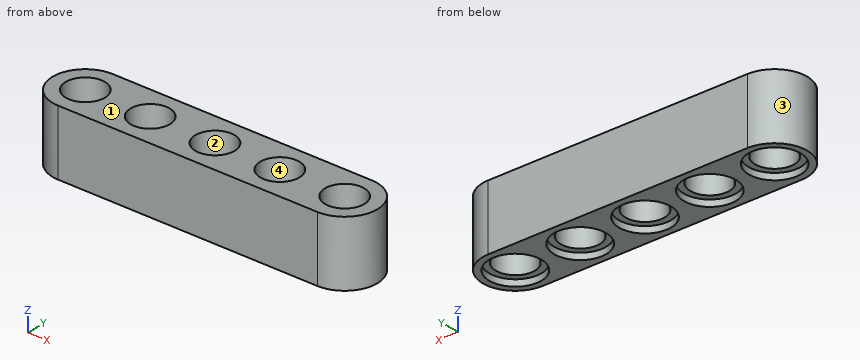
from build123d import *

# Parameters (mm, degrees)
SKETCH_R     = 2.4
PAD_DEPTH    = 8
SKETCH001_R  = 3.2
POCKET_DEPTH = 0.8


with BuildPart() as part:
    # Sketch → Pad (new body)
    with BuildSketch(Plane.XY):
        with BuildLine():
            ThreePointArc((-16, 4), (-20, 0), (-16, -4))
            Line((-16, -4), (16, -4))
            ThreePointArc((16, -4), (20, 0), (16, 4))
            Line((16, 4), (-16, 4))
        make_face()
        with Locations((-16, 0)):
            Circle(SKETCH_R, mode=Mode.SUBTRACT)
        with Locations((16, 0)):
            Circle(SKETCH_R, mode=Mode.SUBTRACT)
        with Locations((8, 0)):
            Circle(SKETCH_R, mode=Mode.SUBTRACT)
        with Locations((-8, 0)):
            Circle(SKETCH_R, mode=Mode.SUBTRACT)
        Circle(SKETCH_R, mode=Mode.SUBTRACT)
    extrude(amount=PAD_DEPTH)

    # Sketch001 → Pocket (cut)
    with BuildSketch(Plane.XY):
        Circle(SKETCH001_R)
        with Locations((-16, 0)):
            Circle(SKETCH001_R)
        with Locations((-8, 0)):
            Circle(SKETCH001_R)
        with Locations((8, 0)):
            Circle(SKETCH001_R)
        with Locations((16, 0)):
            Circle(SKETCH001_R)
    extrude(amount=POCKET_DEPTH, mode=Mode.SUBTRACT)


solid = part.part
Design review of the part built by this model. Coordinates are the model's own, in mm. Face numbers are marked on the shaded views. Round coordinates to 2 decimals unless told otherwise and drop trailing zeros. Write each loop counter-clockwise with the first axis right and the second up, starting at its lowest first coordinate (ties: lowest second). Pieces come first, ordered by that corner, then holes.
Item 1: For pin 1 Ø1.9 at (x, y) = (16, 1.5) entering from -Z; pin 2 Ø3 at (x, y) = (9.5, 1.5) entering from -Z, all flat-tipped, find the tip position at first contact; note any pin that passes through.
Item 2: Wall thickness on L1, parallel to X at y = 0, z = 3.25; L2, parallel to Y at x = 16, z = 4.5; L3, parallel to X at y = 0.5, z = 6.75: over which ranges is each line inside the solid? List them lowest first.
Item 3: Consider section B-B on z = 3.25. Give the boundary of the cut face in (x, y).
Item 4: Consider section A-A on x = 0. Give the boundary of the cut face in (y, z), and give its area (3 significant figures).
Item 5: Consider section D-D on x = 17.5. Give the boundary of the cut face in (y, z).
Item 6: Consider section C-C on y = 0. Count the separate pieces of the cut face and the enclosed holes in it, and give its area (3 significant figures).
Item 7: Draft analysis for pull direction Y (two halves, no side actions). For the marked faces 1, 2, 3 and 4, state which applies: released by +Y, released by -Y, zero draft, split by the parting line, or undercut.
Check values:
1. pin 1: stops at z = 0.8
1. pin 2: stops at z = 0
2. L1: x = -20 to -18.4, -13.6 to -10.4, -5.6 to -2.4, 2.4 to 5.6, 10.4 to 13.6, 18.4 to 20
2. L2: y = -4 to -2.4, 2.4 to 4
2. L3: x = -19.97 to -18.35, -13.65 to -10.35, -5.65 to -2.35, 2.35 to 5.65, 10.35 to 13.65, 18.35 to 19.97
3. outline: (-16, -4) - (16, -4) arc R4 ccw to (16, 4) - (-16, 4) arc R4 ccw to start; hole circle Ø4.8 at (-16, 0); hole circle Ø4.8 at (-8, 0); hole circle Ø4.8 at (0, 0); hole circle Ø4.8 at (8, 0); hole circle Ø4.8 at (16, 0)
4. outline: (-4, 0) - (-3.2, 0) - (-3.2, 0.8) - (-2.4, 0.8) - (-2.4, 8) - (-4, 8) - close; (2.4, 0.8) - (3.2, 0.8) - (3.2, 0) - (4, 0) - (4, 8) - (2.4, 8) - close
4. area: 24.3 mm2
5. outline: (-3.71, 0) - (-2.83, 0) - (-2.83, 0.8) - (-1.87, 0.8) - (-1.87, 8) - (-3.71, 8) - close; (1.87, 0.8) - (2.83, 0.8) - (2.83, 0) - (3.71, 0) - (3.71, 8) - (1.87, 8) - close
6. separate pieces: 6
6. enclosed holes: 0
6. area: 122 mm2
7. face 1: zero draft
7. face 2: undercut
7. face 3: split by the parting line
7. face 4: undercut
